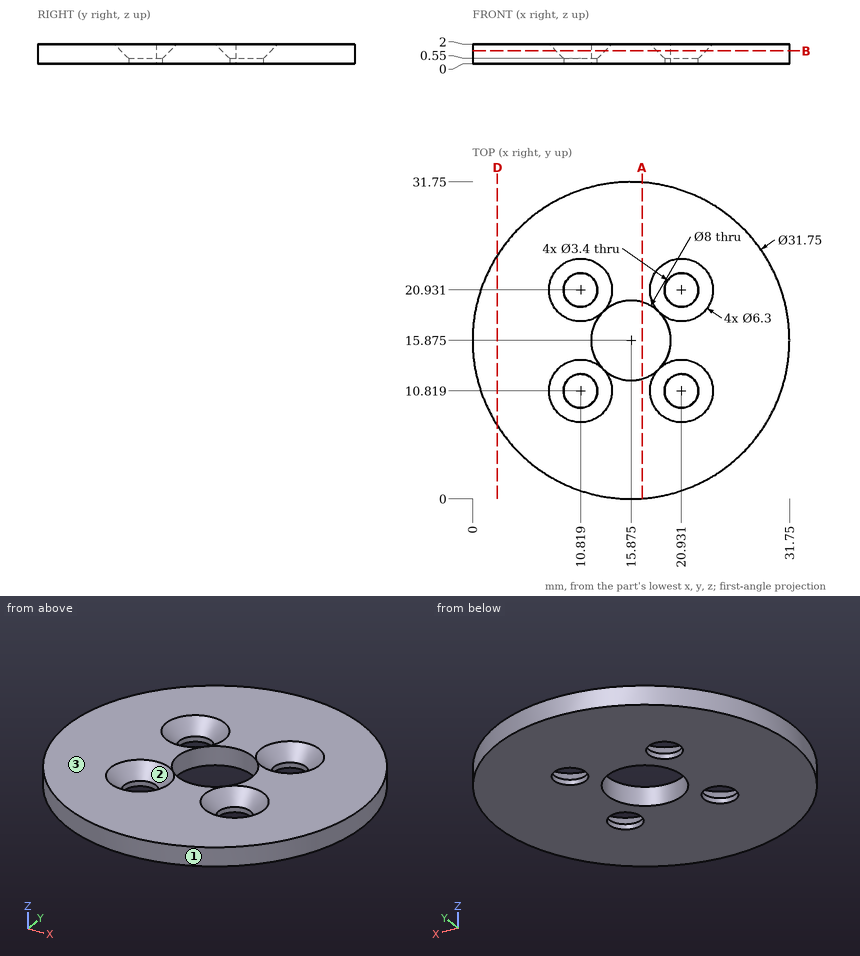
Geometry check sheet. Reference: drawing and pictorial views, mm from the part's lowest x, y, z. Round coordinates to 2 decimals unless told otherwise and drop trailing zeros. Write each loop counter-clockwise with the first axis right and the second up, starting at its lowest first coordinate (ties: lowest second). Pieces come first, ordered by that corner, then holes. Notation, with made-up numbers: (-34.5, -5.5) -> (-16.5, -5.5) arc R6 ccw to (-16.5, 3.5) -> close; hole circle Ø7 at (-26, 33). An arc over 180 degrees is marked (long way). One line per question, with ' | ' between items. Start each with the question number.
1. Sectioned sample at A-A, the plane x = 17. Record the cut outline in (y, z), then the cut area to 3 significant figures.
2. Release check for a two-part mould opening along Y. For the marked faces 1, 2 and 3 record: +Y half, -Y half, draft (parallel to the pull), parting line (faces both ways), or undercut.
3. Scan lines: line 1 along Y through (x, z) = (19, 1) (1 decimal); line 2 along Y through (x, z) = (10.5, 1.05) (1 decimal); line 3 along X through (y, z) = (19.5, 1.7) (1 decimal). Record each from-to range of solid material in increasing order. Write a range as from..to.
4. Sectioned sample at D-D, the plane x = 2.5. Record the cut outline in (y, z), then the cut area to 3 significant figures.
5. Sectioned sample at B-B, the plane z = 1.3. Count the separate pieces of the cut face and the enclosed holes in it, then the cut area to 3 significant figures.
6. Depth check by flat-ended pin: pin 1 (3 mm diameter, centred on x = 27, y = 25.5, fed in from -Z); pin 2 (4 mm diameter, centred on x = 10.82, y = 20.93, fed in from +Z). Enter the tip coordinate at first touch or a pass-through.
Taken from the geometry:
1) outline: (0.04, 0) -> (12.04, 0) -> (12.04, 2) -> (0.04, 2) -> close; (19.71, 0) -> (31.71, 0) -> (31.71, 2) -> (19.71, 2) -> close | area: 48.0 mm^2
2) face 1: parting line | face 2: undercut | face 3: draft
3) line 1: y = 0.3..9.9, 11.8..13.4, 18.4..20, 21.9..31.4 | line 2: y = 0.9..8.6, 13..18.8, 23.1..30.8 | line 3: x = 0.4..8.4, 13.3..14.2, 17.6..18.5, 23.4..31.3
4) outline: (7.32, 0) -> (24.43, 0) -> (24.43, 2) -> (7.32, 2) -> close | area: 34.2 mm^2
5) separate pieces: 1 | enclosed holes: 5 | area: 666 mm^2
6) pin 1: stops at z = 0 | pin 2: stops at z = 0.85
